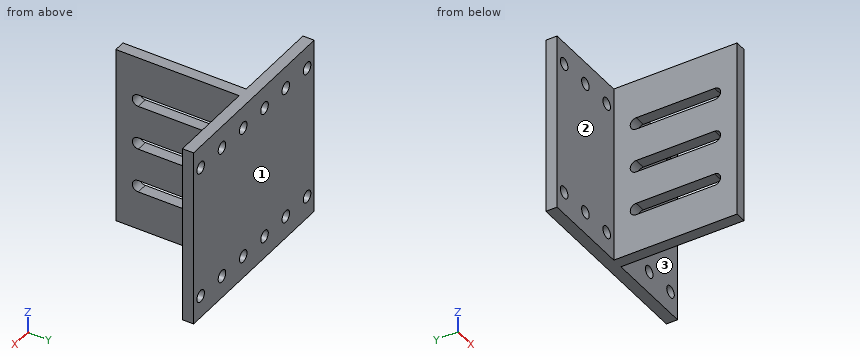
Autodesk Inventor part; units mm, degrees
ref_plane "YZ Plane" through (0, 0, 0) normal (1, 0, 0) x (0, 1, 0)
ref_plane "XZ Plane" through (0, 0, 0) normal (0, 1, 0) x (-1, 0, 0)
ref_plane "XY Plane" through (0, 0, 0) normal (0, 0, 1) x (1, 0, 0)
sketch "Sketch1" plane through (0, 0, 0) normal (0, 1, 0) x (-1, 0, 0)
  line L0 (11.2547, 50.8) -> (-11.2547, 50.8)
  line L1 (-11.2547, 50.8) -> (-11.2547, -50.8)
  line L2 (-11.2547, -50.8) -> (11.2547, -50.8)
  line L3 (11.2547, -50.8) -> (11.2547, 50.8)
  line L4 (11.2547, 50.8) -> (-11.2547, -50.8) construction
  line L5 (-11.2547, 50.8) -> (11.2547, -50.8) construction
  point P0 (0, 0)
  dimension "d0" = 101.6
  dimension "d1" = 22.5095
extrude "Extrusion1" add sketch "Sketch1" against normal blind 6.35
sketch "Sketch2" plane through (0, 0, 0) normal (0, 1, 0) x (1, 0, 0)
  line L0 (11.2547, -50.8) -> (-11.2547, -50.8)
  line L1 (-11.2547, 50.8) -> (11.2547, 50.8)
  line L2 (-11.2547, -50.8) -> (-4.9047, -50.8)
  line L3 (-4.9047, -50.8) -> (-4.9047, 50.8)
  line L4 (-4.9047, 50.8) -> (-11.2547, 50.8)
  line L5 (-11.2547, 50.8) -> (-11.2547, -50.8)
  point P0 (0, 0)
  dimension "d4" = 6.35
extrude "Extrusion2" add sketch "Sketch2" along normal blind 76.2
sketch "Sketch3" plane through (0, 76.2, 0) normal (0, 1, 0) x (1, 0, 0)
  line L0 (11.2547, -50.8) -> (-11.2547, -50.8)
  line L1 (-11.2547, -50.8) -> (-62.0547, -50.8)
  line L2 (-62.0547, -50.8) -> (-62.0547, 50.8)
  line L3 (-62.0547, 50.8) -> (-11.2547, 50.8)
  line L4 (-11.2547, 50.8) -> (-11.2547, -50.8)
  line L5 (-4.9047, -50.8) -> (-4.9047, 50.8)
  line L6 (-4.9047, 50.8) -> (-11.2547, 50.8)
  line L7 (-11.2547, -50.8) -> (-4.9047, -50.8)
  line L8 (11.2547, -50.8) -> (11.2547, 50.8)
  line L9 (11.2547, 50.8) -> (-4.9047, 50.8)
  line L10 (-11.2547, -50.8) -> (-11.2547, 50.8)
  line L11 (-11.2547, -50.8) -> (-4.9047, -50.8)
  line L12 (-4.9047, -50.8) -> (-4.9047, 50.8)
  line L13 (-4.9047, 50.8) -> (-11.2547, 50.8)
  line L14 (-11.2547, 50.8) -> (-11.2547, -50.8)
  line L15 (-4.9047, -50.8) -> (45.8953, -50.8)
  line L16 (45.8953, -50.8) -> (45.8953, 50.8)
  line L17 (45.8953, 50.8) -> (-4.9047, 50.8)
  line L18 (-4.9047, 50.8) -> (-4.9047, -50.8)
  point P0 (0, 0)
  dimension "d7" = 50.8
  dimension "d8" = 50.8
extrude "Extrusion3" add sketch "Sketch3" along normal blind 6.35
sketch "Sketch4" plane through (0, 0, 0) normal (0, 1, 0) x (1, 0, 0)
  line L0 (-4.9047, -50.8) -> (11.2547, -50.8) construction
  line L1 (3.175, -50.8) -> (3.175, 50.8) construction
  line L2 (-11.2547, 50.8) -> (11.2547, 50.8) construction
  point P0 (0, 0)
  point P1 (3.175, -38.1)
  point P2 (3.175, -12.7)
  point P3 (3.175, 12.7)
  point P4 (3.175, 38.1)
  dimension "d11" = 12.7
  dimension "d14" = 25.4
hole "Hole1" at (3.175, 0, 38.1) at (3.175, 0, 12.7) at (3.175, 0, -12.7) at (3.175, 0, -38.1) direction (0, -1, 0) diameter 5.1054 end through all
sketch "Sketch5" plane through (0, 82.55, 0) normal (0, 1, 0) x (1, 0, 0)
  line L0 (-62.0547, 50.8) -> (-62.0547, -50.8) construction
  line L1 (-62.0547, -38.1) -> (42.9055, -38.1) construction
  line L2 (-55.7047, -38.1) -> (-55.7047, 38.1) construction
  point P0 (0, 0)
  point P1 (-36.6547, -38.1)
  point P2 (-36.6547, 38.1)
  point P3 (-17.6047, -38.1)
  point P4 (-17.6047, 38.1)
  point P5 (1.4453, -38.1)
  point P6 (1.4453, 38.1)
  point P7 (20.4953, -38.1)
  point P8 (20.4953, 38.1)
  point P9 (39.5453, -38.1)
  point P10 (39.5453, 38.1)
  point P11 (58.5953, -38.1)
  point P12 (58.5953, 38.1)
  dimension "d26" = 38.1
  dimension "d27" = 76.2
  dimension "d28" = 6.35
  dimension "d31" = 76.2
  dimension "d34" = 19.05
hole "Hole2" at (-55.7047, 82.55, 38.1) at (-55.7047, 82.55, -38.1) at (-36.6547, 82.55, 38.1) at (-36.6547, 82.55, -38.1) at (-17.6047, 82.55, 38.1) at (-17.6047, 82.55, -38.1) at (1.4453, 82.55, 38.1) at (1.4453, 82.55, -38.1) at (20.4953, 82.55, 38.1) at (20.4953, 82.55, -38.1) at (39.5453, 82.55, 38.1) at (39.5453, 82.55, -38.1) at (58.5953, 82.55, 38.1) at (58.5953, 82.55, -38.1) direction (0, -1, 0) diameter 6.7564 depth 6.35
sketch "Sketch8" plane through (11.2547, 0, 50.8) normal (1, 0, 0) x (0, 0, -1)
  line L0 (101.6, -6.35) -> (0, -6.35)
  line L1 (0, 0) -> (0, 76.2)
  line L2 (101.6, 0) -> (101.6, 76.2)
  line L3 (101.6, 0) -> (101.6, -6.35)
  line L4 (0, 0) -> (0, -6.35)
  line L5 (0, -6.35) -> (101.6, -6.35)
  line L6 (101.6, -6.35) -> (101.6, 6.35)
  line L7 (101.6, 6.35) -> (0, 6.35)
  line L8 (0, 6.35) -> (0, -6.35)
  point P0 (50.8, 0)
  point P1 (0, 6.35)
  dimension "d48" = 12.7
extrude "Extrusion5" cut sketch "Sketch8" against normal through all
sketch "Sketch9" plane through (-4.9047, 76.2, 50.8) normal (1, 0, 0) x (0, 0, -1)
  line L0 (101.6, 0) -> (0, 0)
  line L1 (101.6, -69.85) -> (101.6, 0)
  line L2 (101.6, -69.85) -> (0, -69.85)
  line L3 (0, -69.85) -> (0, 0)
  line L4 (0, -12.7) -> (101.6, -12.7) construction
  line L5 (0, -57.15) -> (101.6, -57.15) construction
  line L6 (25.4, -12.7) -> (25.4, -57.15) construction
  line L7 (22.0218, -12.7) -> (22.0218, -57.15)
  line L8 (28.7782, -57.15) -> (28.7782, -12.7)
  arc A0 (28.7782, -12.7) -> (22.0218, -12.7) centre (25.4, -12.7) ccw
  arc A1 (22.0218, -57.15) -> (28.7782, -57.15) centre (25.4, -57.15) ccw
  line L9 (50.8, -12.7) -> (50.8, -57.15) construction
  line L10 (47.4218, -12.7) -> (47.4218, -57.15)
  line L11 (54.1782, -57.15) -> (54.1782, -12.7)
  arc A2 (54.1782, -12.7) -> (47.4218, -12.7) centre (50.8, -12.7) ccw
  arc A3 (47.4218, -57.15) -> (54.1782, -57.15) centre (50.8, -57.15) ccw
  line L12 (76.2, -12.7) -> (76.2, -57.15) construction
  line L13 (72.8218, -12.7) -> (72.8218, -57.15)
  line L14 (79.5782, -57.15) -> (79.5782, -12.7)
  arc A4 (79.5782, -12.7) -> (72.8218, -12.7) centre (76.2, -12.7) ccw
  arc A5 (72.8218, -57.15) -> (79.5782, -57.15) centre (76.2, -57.15) ccw
  point P0 (50.8, -76.2)
  point P1 (25.4, -34.925)
  point P2 (50.8, -34.925)
  point P3 (76.2, -34.925)
  dimension "d51" = 12.7
  dimension "d52" = 12.7
  dimension "d53" = 25.4
  dimension "d54" = 25.4
  dimension "d55" = 25.4
  dimension "d56" = 3.3782
extrude "Extrusion6" cut sketch "Sketch9" against normal through all contours A0 L8 A1 L7 | A2 L11 A3 L10 | A4 L14 A5 L13
equation "\"d0\" = BaseLength"
equation "\"d1\" = BaseWidth"
equation "\"d2\" = BaseThickness"
equation "\"d4\" = BackWidth"
equation "\"d5\" = BackHeight"
equation "\"d7\" = TopBackExtension"
equation "\"d8\" = TopFrontExtension"
equation "\"d9\" = TopThickness"
equation "\"d27\" = holeSpacingForMotorBracket"
equation "\"d28\" = offsetForBracketHoleFromEdge"
equation "\"BaseWidth\" = 22.50948"
equation "\"BaseLength\" = 101.6"
equation "\"BaseThickness\" = 6.35"
equation "\"BackWidth\" = 6.35"
equation "\"BackHeight\" = 76.2"
equation "\"TopBackExtension\" = 50.8"
equation "\"TopFrontExtension\" = 50.8"
equation "\"TopThickness\" = 6.35"
equation "\"offsetForFirstHole\" = 12.7"
equation "\"holeSpacingForMotorBracket\" = 76.2"
equation "\"offsetForBracketHoleFromEdge\" = 6.35"
equation "\"holeSpacingForVariationInMotorBracketHoles\" = 19.05"
equation "\"deltaForSlots\" = 0.25 * BaseLength"
properties part number "pullyBracketTopPortion" material "PC/ABS Plastic"
Check sheet for the modelled part. Datum: model origin and axes. Units: mm. Face numbers are marked on the shaded views. A direction names the side the tool comes from. Coordinates: 2 decimals unless noted, no trailing zeros. Write each loop counter-clockwise with the first axis right and the second up, starting at its lowest first coordinate (ties: lowest second). Pieces come first, ordered by that corner, then holes. Notation, with made-up numbers: (-39, 58.5) -> (5, 58.5) arc R18 ccw to (5, 76.5) -> close; hole circle Ø5 at (-17.5, 17.5). An arc over 180 degrees is marked (long way). Use a Markdown table: item, result.
1. Sectioned sample at C-C (z = -38.1). Give the number of separate pieces and of enclosed holes in the cut face, plus the area to 3 significant figures.
Reported:
| item | result |
|---|---|
| separate pieces | 7 |
| enclosed holes | 0 |
| area | 872 mm2 |
2. Sectioned sample at B-B (z = 0). Enter the section's corners in (x, y).
Reported:
| item | result |
|---|---|
| outline | (-62.05, 76.2) -> (-11.25, 76.2) -> (-11.25, 66.88) -> (-4.9, 66.88) -> (-4.9, 76.2) -> (45.9, 76.2) -> (45.9, 82.55) -> (-62.05, 82.55) -> close; (-11.25, 6.35) -> (-4.9, 6.35) -> (-4.9, 15.67) -> (-11.25, 15.67) -> close |
3. Sectioned sample at D-D (z = 18). Enter the section's corners in (x, y), plus the area to 3 significant figures.
Reported:
| item | result |
|---|---|
| outline | (-62.05, 76.2) -> (-11.25, 76.2) -> (-11.25, 6.35) -> (-4.9, 6.35) -> (-4.9, 76.2) -> (45.9, 76.2) -> (45.9, 82.55) -> (-62.05, 82.55) -> close |
| area | 1,130 mm2 |
4. Tool access check on the marked faces 1, 2 and 3. Record the directions out of +Z, -Z, +X, -X, +Y, -Y that give a thin tool (end or side, any length) a straight path to the whole face; none if there is none.
Reported:
| item | result |
|---|---|
| face 1 | +Z, -Z, +X, -X, +Y |
| face 2 | +Z, -Z, -X, -Y |
| face 3 | +Z, -Z, +X, -Y |
5. Go/stop test with flat-tipped pins: pin 1 Ø1.5 at (y, z) = (47.5, -3) entering from -X; pin 2 Ø10 at (x, z) = (-40, 23.5) entering from -Y; pin 3 Ø1.5 at (y, z) = (24.5, -40.5) entering from +X. Record where each tip stops, or that it passes through.
Reported:
| item | result |
|---|---|
| pin 1 | stops at x = -11.25 |
| pin 2 | stops at y = 76.2 |
| pin 3 | stops at x = -4.9 |
6. Scan lines: line 1 along Z through (x, y) = (-9, 16); line 2 along Y through (x, z) = (-2, 17.5); line 3 along X through (y, z) = (59, -18.5). Record each from-to range of solid material in increasing order.
Reported:
| item | result |
|---|---|
| line 1 | z = -50.8 to -26.85, -23.95 to -1.45, 1.45 to 23.95, 26.85 to 50.8 |
| line 2 | y = 76.2 to 82.55 |
| line 3 | x = -11.25 to -4.9 |
7. Sectioned sample at A-A (y = 42). Enter the section's corners in (x, z), plus the area to 3 significant figures.
Reported:
| item | result |
|---|---|
| outline | (-11.25, -50.8) -> (-4.9, -50.8) -> (-4.9, -28.78) -> (-11.25, -28.78) -> close; (-11.25, -22.02) -> (-4.9, -22.02) -> (-4.9, -3.38) -> (-11.25, -3.38) -> close; (-11.25, 3.38) -> (-4.9, 3.38) -> (-4.9, 22.02) -> (-11.25, 22.02) -> close; (-11.25, 28.78) -> (-4.9, 28.78) -> (-4.9, 50.8) -> (-11.25, 50.8) -> close |
| area | 516 mm2 |
